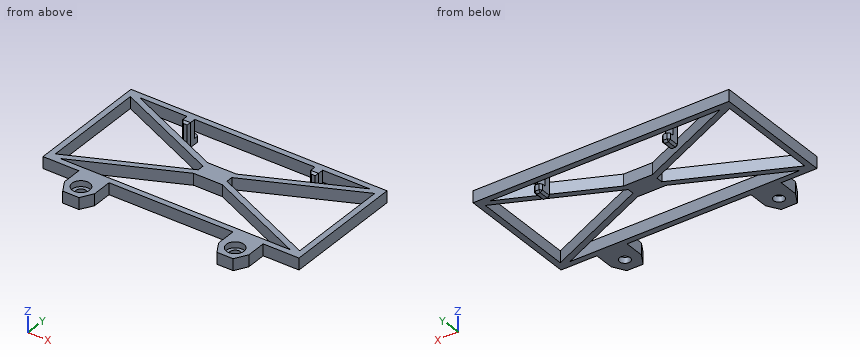
from build123d import *

# Parameters (mm, degrees)
SKETCH1_W                = 66
SKETCH1_H                = 31.5
BOSS_EXTRUDE1_DEPTH      = 3
SKETCH2_R                = 1.375
BOSS_EXTRUDE2_DEPTH      = 3
SKETCH2_4_R              = 2.275
SKETCH2_4_R_2            = 1.375
CUT_EXTRUDE1_DEPTH       = 1.5
BOSS_EXTRUDE3_DEPTH      = 1
CHAMFER1_SIZE            = 0.5
CHAMFER1_OF_MIRROR2_SIZE = 0.5


with BuildPart() as part:
    # Sketch1 → Boss-Extrude1 (new body)
    with BuildSketch(Plane.XY):
        with Locations((0, 0.125155984)):
            Rectangle(SKETCH1_W, SKETCH1_H)
        Polygon((3.706668857, -2.374844016), (29.680353068, -14.124844016), (-29.680353068, -14.124844016), (-3.706668857, -2.374844016), align=None, mode=Mode.SUBTRACT)
        Polygon((-3.706668857, -0.728496791), (-31.5, -13.301670403), (-31.5, 13.551982372), (-3.706668857, 0.97880876), align=None, mode=Mode.SUBTRACT)
        Polygon((-3.706668857, 2.625155984), (-29.680353068, 14.375155984), (29.680353068, 14.375155984), (3.706668857, 2.625155984), align=None, mode=Mode.SUBTRACT)
        Polygon((3.706668857, 0.97880876), (31.5, 13.551982372), (31.5, -13.301670403), (3.706668857, -0.728496791), align=None, mode=Mode.SUBTRACT)
    extrude(amount=BOSS_EXTRUDE1_DEPTH)

    # Sketch2 → Boss-Extrude2 (add)
    with BuildSketch(Plane.XY.offset(3)):
        Polygon((-15.977885683, -15.624844016), (-23.772114317, -15.624844016), (-23.772114317, -20.749844016), (-21.967894726, -23.874844016), (-17.782105274, -23.874844016), (-15.977885683, -20.749844016), align=None)
        with Locations((-19.875, -20.249844016)):
            Circle(SKETCH2_R, mode=Mode.SUBTRACT)
    boss_extrude2 = extrude(amount=-BOSS_EXTRUDE2_DEPTH)

    # Sketch2<4> → Cut-Extrude1 (cut)
    with BuildSketch(Plane.XY.offset(3)):
        with Locations((-19.875, -20.249844016)):
            Circle(SKETCH2_4_R)
        with Locations((-19.875, -20.249844016)):
            Circle(SKETCH2_4_R_2, mode=Mode.SUBTRACT)
    cut_extrude1 = extrude(amount=-CUT_EXTRUDE1_DEPTH, mode=Mode.SUBTRACT)

    # Mirror1: Boss-Extrude2, Cut-Extrude1 across plane
    add(boss_extrude2.mirror(Plane.ZY))
    add(cut_extrude1.mirror(Plane.ZY), mode=Mode.SUBTRACT)

    # Sketch3 → Boss-Extrude3 (add, symmetric)
    with BuildSketch(Plane.ZY.offset(16.5)):
        Polygon((-1.75, 14.375155984), (3, 14.375155984), (3, 12.375155984), (-3.75, 12.375155984), (-3.75, 15.875155984), (-1.75, 15.875155984), align=None)
    boss_extrude3 = extrude(amount=BOSS_EXTRUDE3_DEPTH, both=True)

    # Chamfer1
    chamfer1_edges = [part.edges().sort_by_distance(p)[0] for p in [
        (-16.5, 12.375155984, 3),
        (-15.5, 15.875155984, -2.75),
        (-15.5, 14.125155984, -3.75),
        (-16.5, 15.875155984, -3.75),
        (-15.5, 12.375155984, -0.375),
        (-16.5, 12.375155984, -3.75),
        (-17.5, 15.875155984, -2.75),
        (-17.5, 14.125155984, -3.75),
        (-17.5, 12.375155984, -0.375),
    ]]
    chamfer(chamfer1_edges, length=CHAMFER1_SIZE)

    # Mirror2: Boss-Extrude3 across plane
    add(boss_extrude3.mirror(Plane.ZY))

    # Chamfer1 of Mirror2
    chamfer1_of_mirror2_edges = [part.edges().sort_by_distance(p)[0] for p in [
        (16.5, 12.375155984, 3),
        (15.5, 15.875155984, -2.75),
        (15.5, 14.125155984, -3.75),
        (16.5, 15.875155984, -3.75),
        (15.5, 12.375155984, -0.375),
        (16.5, 12.375155984, -3.75),
        (17.5, 15.875155984, -2.75),
        (17.5, 14.125155984, -3.75),
        (17.5, 12.375155984, -0.375),
    ]]
    chamfer(chamfer1_of_mirror2_edges, length=CHAMFER1_OF_MIRROR2_SIZE)


solid = part.part
The model under review builds one solid part; all positions refer to its coordinate system, in mm. Give positions to 0.01 mm unless a question says otherwise; leave off trailing zeros. Loops run counter-clockwise (first coordinate to the right, second up) from the corner with the lowest first, then second, coordinate; pieces in that order, holes last. Notation, with made-up numbers: (38.25, 27.25) -> (52.25, 27.25) arc R18 cw to (52.25, 31.25) -> close; hole circle Ø4 at (65, 41). An arc over 180 degrees is marked (long way). Put each result on its own line as item: value. Start each with the question number.
1. We need section C-C on y = -17. State the section outline as (x, z) points.
2. Clearance check with flat-ended pins moving along their axes: P1, Ø8, axis at x = 26.5, y = 5.5, coming from the -Z side; P2, Ø1.5, axis at y = -18.5, z = 2, coming from the +X side; P3, Ø6, axis at x = 19.88, y = -20.25, coming from the -Z side; P4, Ø3.5, axis at x = 30.5, z = 1, coming from the -Y side. State where each tip first meets the part, or that it passes through.
3. We need section D-D on y = -4. State the section outline as (x, z) points.
4. Wall thickness on probe 1 along Y at (x, z) = (-9.5, 2.25); probe 2 along X at (y, z) = (-16.5, 2); probe 3 along X at (y, z) = (7.5, 0.75): over which ranges is each line inside the solid? List them lowest first.
5. We need section A-A on y = 0. State the section outline as (x, z) points, then the cut area to 3 significant figures.
6. We need section B-B on x = 3. State the section outline as (y, z) points.
Determined:
1. outline: (-23.77, 0) -> (-15.98, 0) -> (-15.98, 3) -> (-23.77, 3) -> close; (15.98, 0) -> (23.77, 0) -> (23.77, 3) -> (15.98, 3) -> close
2. P1: through
2. P2: x = 23.77
2. P3: z = 0
2. P4: y = -15.62
3. outline: (-33, 0) -> (-31.5, 0) -> (-31.5, 3) -> (-33, 3) -> close; (-10.94, 0) -> (-7.3, 0) -> (-7.3, 3) -> (-10.94, 3) -> close; (7.3, 0) -> (10.94, 0) -> (10.94, 3) -> (7.3, 3) -> close; (31.5, 0) -> (33, 0) -> (33, 3) -> (31.5, 3) -> close
4. probe 1: -15.62 to -14.12, -5 to -3.35, 3.6 to 5.25, 14.38 to 15.88
4. probe 2: -23.77 to -15.98, 15.98 to 23.77
4. probe 3: -33 to -31.5, -18.12 to -14.48, 14.48 to 18.12, 31.5 to 33
5. outline: (-33, 0) -> (-31.5, 0) -> (-31.5, 3) -> (-33, 3) -> close; (-3.71, 0) -> (3.71, 0) -> (3.71, 3) -> (-3.71, 3) -> close; (31.5, 0) -> (33, 0) -> (33, 3) -> (31.5, 3) -> close
5. area: 31.2 mm^2
6. outline: (-15.62, 0) -> (-14.12, 0) -> (-14.12, 3) -> (-15.62, 3) -> close; (-2.37, 0) -> (2.63, 0) -> (2.63, 3) -> (-2.37, 3) -> close; (14.38, 0) -> (15.88, 0) -> (15.88, 3) -> (14.38, 3) -> close
